For this review, take the finished solid that the model builds, in its own axes (mm). A direction names the side the tool comes from. Round coordinates to 2 decimals unless told otherwise and drop trailing zeros. Order: outer loops, then holes, each group sorted by start corner. A loop starts at its lowest first (then second) coordinate and runs counter-clockwise, first axis right, second up. Notation, with made-up numbers: M -22,-13.75 L 3,-13.75 A23 cw 3,7.25 Z; hole C 75,43 d9. An arc over 180 degrees is marked long. Use a Markdown table: item, result.
from build123d import *

# Parameters (mm, degrees)
SKETCH_W        = 44
SKETCH_H        = 250
PAD_DEPTH       = 15
SKETCH001_R     = 3.25
POCKET_DEPTH    = 15
SKETCH002_R     = 2.75
POCKET001_DEPTH = 15
SKETCH003_R     = 5.2
POCKET002_DEPTH = 6
SKETCH004_R     = 5.2
POCKET003_DEPTH = 15


with BuildPart() as part:
    # Sketch → Pad (new body)
    with BuildSketch(Plane.XY):
        with Locations((22, 125)):
            Rectangle(SKETCH_W, SKETCH_H)
    extrude(amount=PAD_DEPTH)

    # Sketch001 (on Face6 of Pad) → Pocket (cut)
    with BuildSketch(Plane.XY.offset(15)):
        with Locations((22, 230)):
            Circle(SKETCH001_R)
        with Locations((22, 125)):
            Circle(SKETCH001_R)
        with Locations((22, 20)):
            Circle(SKETCH001_R)
    extrude(amount=-POCKET_DEPTH, mode=Mode.SUBTRACT)

    # Sketch002 (on Face5 of Pocket) → Pocket001 (cut)
    with BuildSketch(Plane.XY.offset(15)):
        with Locations((6, 206)):
            Circle(SKETCH002_R)
        with Locations((38, 206)):
            Circle(SKETCH002_R)
        with Locations((6, 170)):
            Circle(SKETCH002_R)
        with Locations((38, 170)):
            Circle(SKETCH002_R)
        with Locations((6, 86)):
            Circle(SKETCH002_R)
        with Locations((38, 86)):
            Circle(SKETCH002_R)
        with Locations((6, 50)):
            Circle(SKETCH002_R)
        with Locations((38, 50)):
            Circle(SKETCH002_R)
    extrude(amount=-POCKET001_DEPTH, mode=Mode.SUBTRACT)

    # Sketch003 (on Face5 of Pocket001) → Pocket002 (cut)
    with BuildSketch(Plane.XY.offset(15)):
        with Locations((22, 20)):
            Circle(SKETCH003_R)
        with Locations((22, 125)):
            Circle(SKETCH003_R)
        with Locations((22, 230)):
            Circle(SKETCH003_R)
    extrude(amount=-POCKET002_DEPTH, mode=Mode.SUBTRACT)

    # Sketch004 (on Face5 of Pocket002) → Pocket003 (cut)
    with BuildSketch(Plane.XY.offset(15)):
        with Locations((22, 188.5)):
            Circle(SKETCH004_R)
    extrude(amount=-POCKET003_DEPTH, mode=Mode.SUBTRACT)


solid = part.part
Q1. Add section A-A (y = 230). Write out the cut boundary in (x, z), then the cut area to 3 significant figures.
Determined:
| item | result |
|---|---|
| outline | M 0,0 L 18.75,0 L 18.75,9 L 16.8,9 L 16.8,15 L 0,15 Z; M 25.25,0 L 44,0 L 44,15 L 27.2,15 L 27.2,9 L 25.25,9 Z |
| area | 539 mm^2 |
Q2. Machinability: for faces 4 (the cylindrical face through (5.642, 52.727, 7.605)), 5 (the flat face through (25.4, 20.1, 9)), which of the approach directions +Z, -Z, +X, -X, +Y, -Y give a long, thin tool a straight path to every point of the face, cutting with its end or side? Answer none if there is none.
Determined:
| item | result |
|---|---|
| face 4 | +Z, -Z |
| face 5 | +Z |
Q3. Clearance check with flat-ended pins moving along their axes: pin 1 (3.5 mm diameter, centred on x = 6, y = 206, fed in from +Z); pin 2 (5 mm diameter, centred on x = 22, y = 22.5, fed in from +Z). State where each tip first meets the part, or that it passes through.
Determined:
| item | result |
|---|---|
| pin 1 | passes through |
| pin 2 | stops at z = 9 |
Q4. Wall thickness on line 1 along Y through (x, z) = (38, 3.75); line 2 along X through (y, z) = (170, 8.75); line 3 along X through (y, z) = (121, 12.75): over which ranges is each line inside the solid? List them lowest first. Write a range as [from, to].
Determined:
| item | result |
|---|---|
| line 1 | y = [0, 47.25], [52.75, 83.25], [88.75, 167.25], [172.75, 203.25], [208.75, 250] |
| line 2 | x = [0, 3.25], [8.75, 35.25], [40.75, 44] |
| line 3 | x = [0, 18.68], [25.32, 44] |
Q5. Add section B-B (x = 38). Write out the cut boundary in (y, z).
Determined:
| item | result |
|---|---|
| outline | M 0,0 L 47.25,0 L 47.25,15 L 0,15 Z; M 52.75,0 L 83.25,0 L 83.25,15 L 52.75,15 Z; M 88.75,0 L 167.25,0 L 167.25,15 L 88.75,15 Z; M 172.75,0 L 203.25,0 L 203.25,15 L 172.75,15 Z; M 208.75,0 L 250,0 L 250,15 L 208.75,15 Z |
Q6. Add section C-C (z = 2.5). Give the number of separate pieces and of enclosed holes in the cut face, then the cut area to 3 significant figures.
Determined:
| item | result |
|---|---|
| separate pieces | 1 |
| enclosed holes | 12 |
| area | 10,600 mm^2 |
Q7. Draft analysis for pull direction X (two halves, no side actions). For faces 1 (the flat face through (25.4, 230.1, 9)), 2 (the flat face through (0, 123, 7)), 3 (the flat face through (22, 0, 7)), state which applies: pulls with the +X half, pulls with the -X half, needs draft (parallel to the pull), parting line crosses it, or undercut.
Determined:
| item | result |
|---|---|
| face 1 | undercut |
| face 2 | pulls with the -X half |
| face 3 | needs draft |
Q8. Add section D-D (y = 170). Write out the cut boundary in (x, z), then the cut area to 3 significant figures.
Determined:
| item | result |
|---|---|
| outline | M 0,0 L 3.25,0 L 3.25,15 L 0,15 Z; M 8.75,0 L 35.25,0 L 35.25,15 L 8.75,15 Z; M 40.75,0 L 44,0 L 44,15 L 40.75,15 Z |
| area | 495 mm^2 |
